Can you work these out from the model? Positions are in its coordinate system, mm. Face numbers are marked on the shaded views. A direction names the side the tool comes from. Give positions to 0.01 mm unless a question says otherwise; leave off trailing zeros. Order: outer loops, then holes, each group sorted by start corner. A loop starts at its lowest first (then second) coordinate and runs counter-clockwise, first axis right, second up. Notation, with made-up numbers: (56.5, -35) - (81.5, -35) arc R17 ccw to (81.5, -5) - close; hole circle Ø9 at (79.25, 75). An arc over 180 degrees is marked (long way). Use one line per item in the form item = value. Start each with the question number.
1) For pin 1 (5 mm diameter, centred on x = -51, z = 10.5, fed in from +Y); pin 2 (4.5 mm diameter, centred on y = 35.5, z = 16, fed in from -X); pin 3 (12 mm diameter, centred on y = -11, z = 17.5, fed in from +X), each with a flat end and sliding along its axis, tell me the tip position at first contact or that it passes through.
2) Suppose I cut it at D-D, the plane y = 33. Write out the boundary of the cut face in (x, z), and give its area (3 significant figures).
3) Suppose I cut it at A-A, the plane x = -15. Write out the boundary of the cut face in (y, z), and give its area (3 significant figures).
4) Suppose I cut it at C-C, the plane y = 0. Write out the boundary of the cut face in (x, z), and give its area (3 significant figures).
5) We'd pull the mould along X, two halves only. Please class the marked faces 1, 2, 3 and 4: released by +X, released by -X, zero draft, split by the parting line, or undercut.
6) Suppose I cut it at B-B, the plane x = -0.6. Write out the boundary of the cut face in (y, z), and give its area (3 significant figures).
7) Which directions (+Z, -Z, +X, -X, +Y, -Y) give clear straight access to the entire face, cutting with the end or side of a thin tool? Please do the marked faces 5, 6 and 7.
8) Please list where these lines run through material, in increasing order: probe 1 along X at (y, z) = (7.5, 17.5); probe 2 along Y at (x, z) = (40, 0.25); probe 3 along Y at (x, z) = (-0.6, 11.5).
```python
from build123d import *

# Parameters (mm, degrees)
SKETCH1_W           = 120
SKETCH1_H           = 80
SKETCH1_R           = 10
SKETCH1_R_2         = 11
BOSS_EXTRUDE1_DEPTH = 3.5
SKETCH2_R           = 17.5
SKETCH2_R_2         = 10
BOSS_EXTRUDE2_DEPTH = 3
SKETCH3_W           = 6
SKETCH3_H           = 20
SKETCH3_R           = 2.25
BOSS_EXTRUDE3_DEPTH = 26.11
CUT_EXTRUDE1_START  = -26.11
SKETCH4_R           = 2.25
CUT_EXTRUDE1_DEPTH  = 26.11
SKETCH5_W           = 30
SKETCH5_H           = 15
BOSS_EXTRUDE4_DEPTH = 30
SKETCH6_R           = 4
CUT_EXTRUDE2_DEPTH  = 29


with BuildPart() as part:
    # Sketch1 → Boss-Extrude1 (new, symmetric)
    with BuildSketch(Plane.XY):
        Rectangle(SKETCH1_W, SKETCH1_H)
        with Locations((-15, 0)):
            Circle(SKETCH1_R, mode=Mode.SUBTRACT)
        with Locations((40, 0)):
            Circle(SKETCH1_R_2, mode=Mode.SUBTRACT)
    extrude(amount=BOSS_EXTRUDE1_DEPTH, both=True)

    # Sketch2 → Boss-Extrude2 (add)
    with BuildSketch(Plane.XY.offset(3.5)):
        with Locations(Location((40, 0, 0), (0, 0, 180))):
            Circle(SKETCH2_R)
        with Locations((40, 0)):
            Circle(SKETCH2_R_2, mode=Mode.SUBTRACT)
    extrude(amount=BOSS_EXTRUDE2_DEPTH)

    # Sketch3 → Boss-Extrude3 (add)
    # profile 1 of 2: a face of its own
    with BuildSketch(Plane.XY.offset(3.5)):
        with Locations((-50, 0)):
            Rectangle(SKETCH3_W, SKETCH3_H)
        with Locations(Location((-50.1, -5, 0), (0, 0, 180))):
            Circle(SKETCH3_R, mode=Mode.SUBTRACT)
        with Locations(Location((-50.1, 5, 0), (0, 0, 180))):
            Circle(SKETCH3_R, mode=Mode.SUBTRACT)
    # profile 2 of 2: a face of its own
    with BuildSketch(Plane.XY.offset(3.5)):
        with Locations((-0.6, 0)):
            Rectangle(SKETCH3_W, SKETCH3_H)
        with Locations(Location((-0.6, -5, 0), (0, 0, 180))):
            Circle(SKETCH3_R, mode=Mode.SUBTRACT)
        with Locations(Location((-0.6, 5, 0), (0, 0, 180))):
            Circle(SKETCH3_R, mode=Mode.SUBTRACT)
    extrude(amount=BOSS_EXTRUDE3_DEPTH)

    # Sketch4 → Cut-Extrude1 (cut)
    with BuildSketch(Plane.XY.offset(3.5).offset(CUT_EXTRUDE1_START)):
        with Locations(Location((-50.1, 5, 0), (0, 0, 180))):
            Circle(SKETCH4_R)
        with Locations(Location((-50.1, -5, 0), (0, 0, 180))):
            Circle(SKETCH4_R)
        with Locations(Location((-0.6, 5, 0), (0, 0, 180))):
            Circle(SKETCH4_R)
        with Locations(Location((-0.6, -5, 0), (0, 0, 180))):
            Circle(SKETCH4_R)
    extrude(amount=CUT_EXTRUDE1_DEPTH, mode=Mode.SUBTRACT)

    # Sketch5 → Boss-Extrude4 (add)
    with BuildSketch(Plane.XY.offset(3.5)):
        with Locations((12.5, 32.5)):
            Rectangle(SKETCH5_W, SKETCH5_H)
    extrude(amount=BOSS_EXTRUDE4_DEPTH)

    # Sketch6 → Cut-Extrude2 (cut)
    with BuildSketch(Plane(origin=(0, 40, 0), x_dir=(1, 0, 0), z_dir=(0, 1, 0))):
        with Locations(Location((12.5, -18.5, 0), (0, 0, 270))):
            Circle(SKETCH6_R)
    extrude(amount=-CUT_EXTRUDE2_DEPTH, mode=Mode.SUBTRACT)


solid = part.part
```
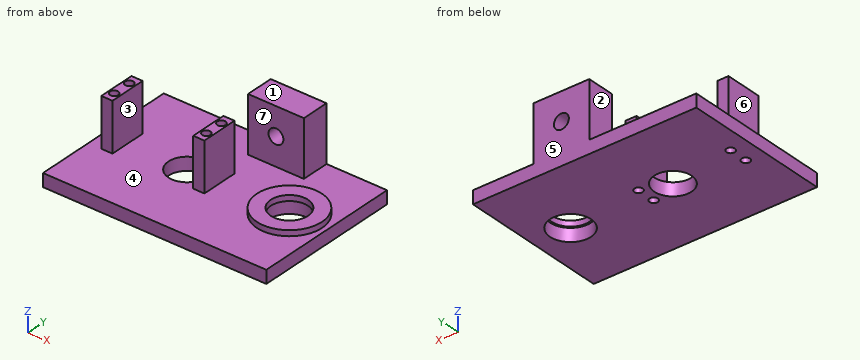
Result sheet:
q1.pin_1 = 10
q1.pin_2 = -2.5
q1.pin_3 = 2.4
q2.outline = (-60, -3.5) - (60, -3.5) - (60, 3.5) - (27.5, 3.5) - (27.5, 33.5) - (-2.5, 33.5) - (-2.5, 3.5) - (-60, 3.5) - close; hole circle Ø8 at (12.5, 18.5)
q2.area = 1,690 mm²
q3.outline = (-40, -3.5) - (-10, -3.5) - (-10, 3.5) - (-40, 3.5) - close; (10, -3.5) - (40, -3.5) - (40, 3.5) - (10, 3.5) - close
q3.area = 420 mm²
q4.outline = (-60, -3.5) - (-25, -3.5) - (-25, 3.5) - (-47, 3.5) - (-47, 29.61) - (-53, 29.61) - (-53, 3.5) - (-60, 3.5) - close; (-5, -3.5) - (29, -3.5) - (29, 3.5) - (30, 3.5) - (30, 6.5) - (22.5, 6.5) - (22.5, 3.5) - (2.4, 3.5) - (2.4, 29.61) - (-3.6, 29.61) - (-3.6, 3.5) - (-5, 3.5) - close; (50, 3.5) - (51, 3.5) - (51, -3.5) - (60, -3.5) - (60, 3.5) - (57.5, 3.5) - (57.5, 6.5) - (50, 6.5) - close
q4.area = 904 mm²
q5.face_1 = zero draft
q5.face_2 = released by -X
q5.face_3 = undercut
q5.face_4 = undercut
q6.outline = (-40, -3.5) - (-7.25, -3.5) - (-7.25, 29.61) - (-10, 29.61) - (-10, 3.5) - (-40, 3.5) - close; (-2.75, -3.5) - (2.75, -3.5) - (2.75, 29.61) - (-2.75, 29.61) - close; (7.25, -3.5) - (40, -3.5) - (40, 33.5) - (25, 33.5) - (25, 3.5) - (10, 3.5) - (10, 29.61) - (7.25, 29.61) - close
q6.area = 1,230 mm²
q7.face_5 = +Z, -Z, +X, -X, +Y
q7.face_6 = +Z, -X, +Y, -Y
q7.face_7 = +Z, +X, -X
q8.probe_1 = -53 to -47, -3.6 to 2.4
q8.probe_2 = -40 to -11, 11 to 40
q8.probe_3 = -10 to -7.25, -2.75 to 2.75, 7.25 to 10, 25 to 40
